Verification items for the finished model (mm, model axes). A direction names the side the tool comes from. Round coordinates to 2 decimals unless told otherwise and drop trailing zeros. Order: outer loops, then holes, each group sorted by start corner. A loop starts at its lowest first (then second) coordinate and runs counter-clockwise, first axis right, second up. Notation, with made-up numbers: M 28,-24.5 L 56,-24.5 A14 cw 56,-11.5 Z; hole C 8.5,-29 d10. An arc over 180 degrees is marked long. One line per item, written item: value. Start each with the question number.
from build123d import *

# Parameters (mm, degrees)
F0_W     = 76.2
F0_H     = 25.4
F1_DEPTH = 5
F2_W     = 76.2
F2_H     = 5
F3_DEPTH = 5
F4_R     = 4.99999
F5_W     = 2
F5_H     = 2
F7_DEPTH = 2
F6_W     = 3
F6_H     = 1
F8_DEPTH = 10.001


# Not quite as in the source:
# - a fillet or chamfer is up to 0.001 mm smaller than in the source, because OpenCascade refuses the exact size


with BuildPart() as f1:
    # F0 (on Top) → F1 (new body)
    with BuildSketch(Plane.XY):
        Rectangle(F0_W, F0_H)
    extrude(amount=F1_DEPTH)

    # F2 (on face) → F3 (join)
    with BuildSketch(Plane.XY.offset(5)):
        Rectangle(F2_W, F2_H)
    extrude(amount=F3_DEPTH)

    # F4 (radius 5 in the source; OpenCascade refuses exactly that, so slightly less here)
    f4_edges = [f1.edges().sort_by_distance(p)[0] for p in [
        (0, -2.5, 5),
        (0, 2.5, 5),
    ]]
    fillet(f4_edges, radius=F4_R)

    # F5 (on face) → F7 (cut)
    with BuildSketch(Plane.XY.offset(10)):
        with Locations((35.1, 0)):
            Rectangle(F5_W, F5_H)
        with Locations((-35.1, 0)):
            Rectangle(F5_W, F5_H)
    extrude(amount=-F7_DEPTH, mode=Mode.SUBTRACT)

    # F6 (on face) → F8 (cut, through all)
    with BuildSketch(Plane.XY.offset(10)):
        with Locations((36.6, 0)):
            Rectangle(F6_W, F6_H)
        with Locations((-36.6, 0)):
            Rectangle(F6_W, F6_H)
    extrude(amount=-F8_DEPTH, mode=Mode.SUBTRACT)


solid = f1.part
1. Section check C-C (z = 8.75). Record the cut outline in (x, y).
2. Scan lines: line 1 along X through (y, z) = (0, 6.75); line 2 along Z through (x, y) = (33, 7.5); line 3 along Z through (x, y) = (-28, 3.5). Record each from-to range of solid material in increasing order.
3. Tool access check on faces 1 (the face through (38.1, -5, 4)), 2 (the face through (-37, 0.5, 5)), 3 (the face through (-35, -1, 9)), 4 (the face through (37, -0.5, 5)), 5 (the face through (-1, -10, 5)). Record the directions out of +Z, -Z, +X, -X, +Y, -Y that give a thin tool (end or side, any length) a straight path to the whole face; none if there is none.
4. Depth check by flat-ended pin: pin 1 (0.8 mm diameter, centred on y = 0, z = 3, fed in from +X); pin 2 (0.6 mm diameter, centred on x = 35, z = 8.5, fed in from +Y); pin 3 (1 mm diameter, centred on x = -34.5, z = 8.5, fed in from +Y). Enter the tip coordinate at first touch or a pass-through.
5. Draft check along X on faces 6 (the face through (-38.1, 5, 4)), 7 (the face through (38.1, 5, 4)), 8 (the face through (-34.9, 0, 8)), 9 (the face through (-37, -0.5, 5)). Enter one of: released by +X, released by -X, zero draft, split by the parting line, or undercut.
6. Section check B-B (y = -4.5). Record the cut outline in (x, z), and give its area (3 significant figures).
7. Section check D-D (y = -8.5). Record the cut outline in (x, z).
Geometry check:
1. outline: M -38.1,-2.66 L 38.1,-2.66 L 38.1,-0.5 L 36.1,-0.5 L 36.1,-1 L 34.1,-1 L 34.1,1 L 36.1,1 L 36.1,0.5 L 38.1,0.5 L 38.1,2.66 L -38.1,2.66 L -38.1,0.5 L -36.1,0.5 L -36.1,1 L -34.1,1 L -34.1,-1 L -36.1,-1 L -36.1,-0.5 L -38.1,-0.5 Z
2. line 1: x = -35.1 to 35.1
2. line 2: z = 0 to 5
2. line 3: z = 0 to 7
3. face 1: +Z, -Z, +X, +Y, -Y
3. face 2: +Z, -Z, -X
3. face 3: +Z
3. face 4: +Z, -Z, +X
3. face 5: +Z, +X, -X, -Y
4. pin 1: stops at x = 35.1
4. pin 2: stops at y = 2.84
4. pin 3: stops at y = 2.92
5. face 6: released by -X
5. face 7: released by +X
5. face 8: undercut
5. face 9: zero draft
6. outline: M -38.1,0 L 38.1,0 L 38.1,6 L -38.1,6 Z
6. area: 457 mm²
7. outline: M -38.1,0 L 38.1,0 L 38.1,5 L -38.1,5 Z
